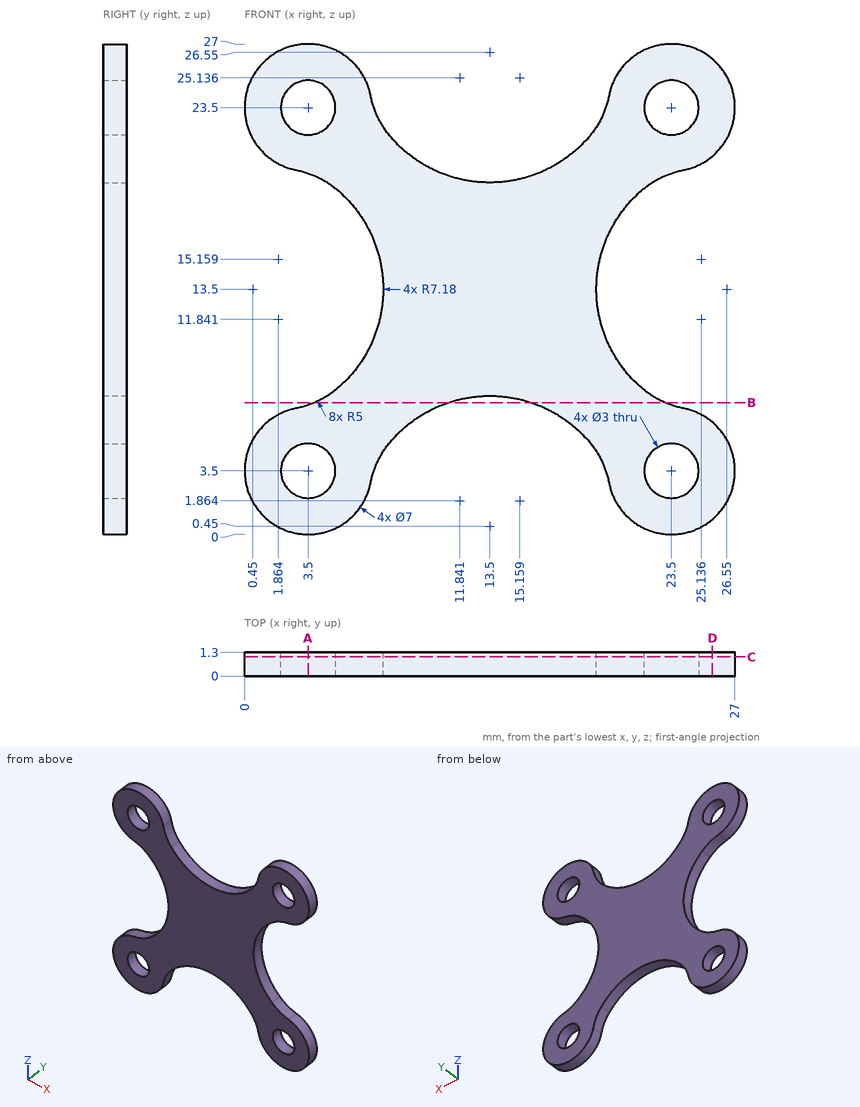
The drawing under review shows one solid part. Ordinate dimensions are in mm from its lowest x, y, z. Round coordinates to 2 decimals unless told otherwise and drop trailing zeros. Write each loop counter-clockwise with the first axis right and the second up, starting at its lowest first coordinate (ties: lowest second). Pieces come first, ordered by that corner, then holes. Notation, with made-up numbers: (-32, 9) -> (17, 9) arc R15 cw to (17, 36) -> close; hole circle Ø7 at (19, 47.5). An arc over 180 degrees is marked (long way). Put each result on its own line as item: value.
Q1. Clearance check with a flat-ended pin moving along its axis: pin 1 Ø2.5 at (x, z) = (23.5, 23.5) entering from -Y. State where the tip first meets the part, or that it passes through.
Determined:
pin 1: passes through
Q2. Consider section C-C on y = 1.05. Give the number of separate pieces and of enclosed holes in the cut face, and give its area (3 significant figures).
Determined:
separate pieces: 1
enclosed holes: 4
area: 334 mm^2
Q3. To check wall thickness, follow L1, parallel to Z at x = 3.5, y = 0.7 (1 decimal); L2, parallel to X at y = 1, z = 24 (1 decimal); L3, parallel to Z at x = 23.75, y = 0.65. State the ranges of each line that lie inside material, in increasing order. Write a range as [from, to].
Determined:
L1: z = [0, 2], [5, 7.1], [19.9, 22], [25, 27]
L2: x = [0, 2.1], [4.9, 7], [20, 22.1], [24.9, 27]
L3: z = [0.01, 2.02], [4.98, 7.04], [19.96, 22.02], [24.98, 26.99]
Q4. Consider section A-A on x = 3.5. State the section outline as (y, z) points.
Determined:
outline: (0, 0) -> (1.3, 0) -> (1.3, 2) -> (0, 2) -> close; (0, 5) -> (1.3, 5) -> (1.3, 7.12) -> (0, 7.12) -> close; (0, 19.88) -> (1.3, 19.88) -> (1.3, 22) -> (0, 22) -> close; (0, 25) -> (1.3, 25) -> (1.3, 27) -> (0, 27) -> close
Q5. Consider section B-B on z = 7.25. State the section outline as (x, y) points (1 decimal).
Determined:
outline: (3.8, 0) -> (11.2, 0) -> (11.2, 1.3) -> (3.8, 1.3) -> close; (15.8, 0) -> (23.2, 0) -> (23.2, 1.3) -> (15.8, 1.3) -> close
Q6. Consider section D-D on x = 25.75. State the section outline as (y, z) points.
Determined:
outline: (0, 0.82) -> (1.3, 0.82) -> (1.3, 6.18) -> (0, 6.18) -> close; (0, 20.82) -> (1.3, 20.82) -> (1.3, 26.18) -> (0, 26.18) -> close
